The drawing under review shows one solid part. Ordinate dimensions are in mm from its lowest x, y, z. A direction names the side the tool comes from. Coordinates: 2 decimals unless noted, no trailing zeros. Write each loop counter-clockwise with the first axis right and the second up, starting at its lowest first coordinate (ties: lowest second). Pieces come first, ordered by that corner, then holes.
Q1. Take a section at C-C (y = 7.5). Give the boundary of the cut face in (x, z), and give its area (3 significant figures).
Q2. Take a section at B-B (z = 67.5). Give the boundary of the cut face in (x, y) (3 decimals).
Q3. For probe 1 along Y at (x, z) = (0.5, 24) (3 decimals); probe 2 along Z at (x, y) = (4.5, 5.5), list the stretches that pass through material, from the lowest coordinate up.
Q4. Take a section at A-A (x = 1). Give the boundary of the cut face in (y, z) (3 decimals).
Q5. Insertion check: pin 1 (1.9 mm diameter, centred on x = 1.5, z = 66, fed in from +Y) (3 decimals); pin 2 (1.9 mm diameter, centred on x = 2.5, y = 42.5, fed in from +Z); pin 3 (3 mm diameter, centred on x = 2, y = 4, fed in from -Z); pin 4 (1.5 mm diameter, centred on x = 3, y = 31.5, fed in from -Z). Each pin has a flat end and moves straight along its axis. Give the tip position at first contact, or say it passes through.
Q6. Machinability: for the marked faces 1, 2, 3, 4 and 5, which of the approach directions +Z, -Z, +X, -X, +Y, -Y give a long, thin tool a straight path to every point of the face, cutting with its end or side? Answer none if there is none.
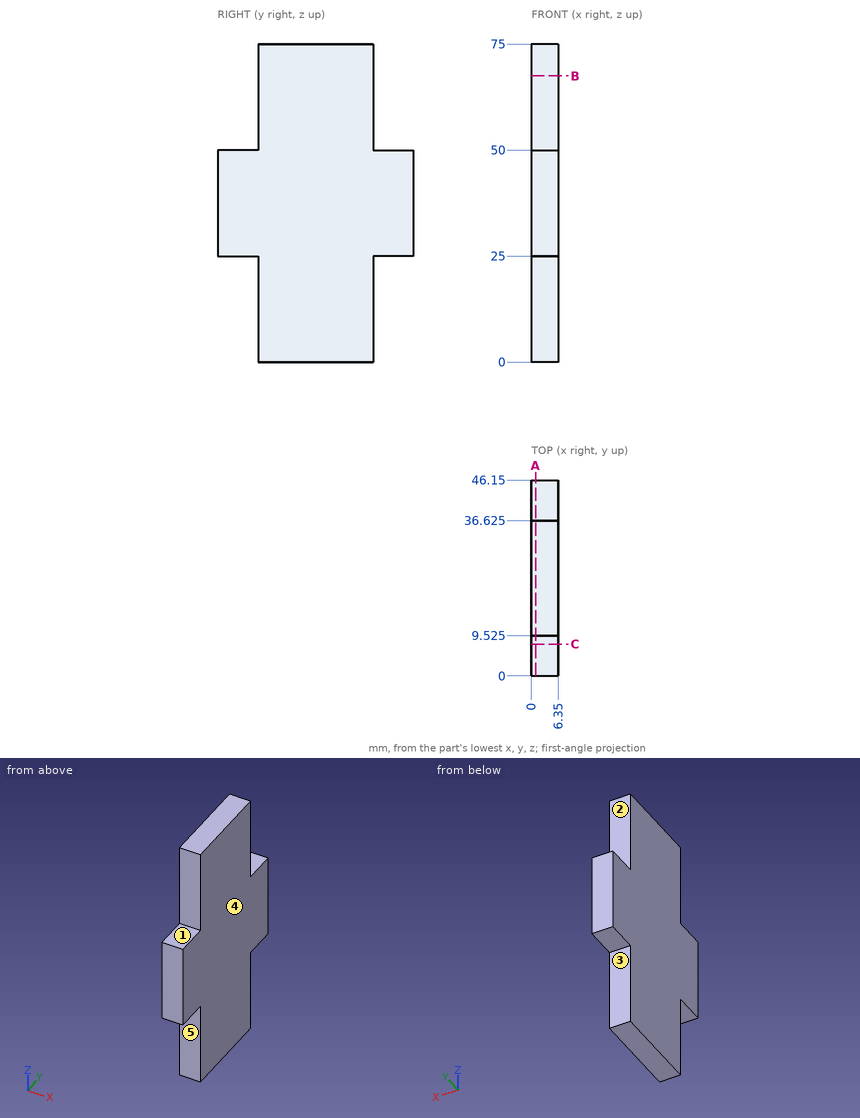
Response:
1. outline: (0, 25) - (6.35, 25) - (6.35, 50) - (0, 50) - close
1. area: 159 mm2
2. outline: (0, 9.525) - (6.35, 9.525) - (6.35, 36.625) - (0, 36.625) - close
3. probe 1: y = 9.525 to 36.625
3. probe 2: z = 25 to 50
4. outline: (0, 25) - (9.525, 25) - (9.525, 0) - (36.625, 0) - (36.625, 25) - (46.15, 25) - (46.15, 50) - (36.625, 50) - (36.625, 75) - (9.525, 75) - (9.525, 50) - (0, 50) - close
5. pin 1: stops at y = 36.625
5. pin 2: stops at z = 50
5. pin 3: stops at z = 25
5. pin 4: stops at z = 0
6. face 1: +Z, +X, -X, -Y
6. face 2: +Z, +X, -X, +Y
6. face 3: -Z, +X, -X, +Y
6. face 4: +Z, -Z, +X, +Y, -Y
6. face 5: -Z, +X, -X, -Y
